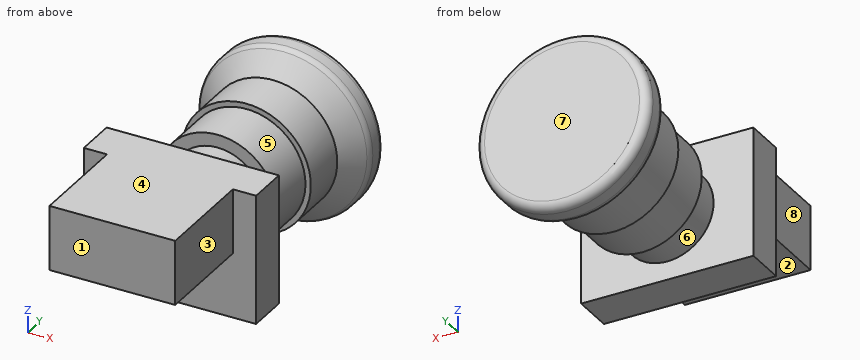
```python
from build123d import *

# Parameters (mm, degrees)
CROQUIS1_W              = 13.75
CROQUIS1_H              = 12
CROQUIS5_R              = 10.75
SALIENTE_EXTRUIR3_DEPTH = 10.3
CROQUIS8_W              = 40
CROQUIS8_H              = 30
SALIENTE_EXTRUIR4_DEPTH = 9.5
CROQUIS9_W              = 29.2
CROQUIS9_H              = 15
SALIENTE_EXTRUIR5_DEPTH = 24


with BuildPart() as part:
    # Croquis1 → Revolución1 (revolve)
    with BuildSketch(Plane.XY, mode=Mode.PRIVATE) as revoluci_n1_sk:
        with Locations((6.875, 6)):
            Rectangle(CROQUIS1_W, CROQUIS1_H)
    revolve(revoluci_n1_sk.sketch.rotate(Axis((0, 0, 0), (0, 1, 0)), 90), axis=Axis((0, 0, 0), (0, 1, 0)))

    # Croquis2 → Revolución2 (revolve)
    with BuildSketch(Plane.XY, mode=Mode.PRIVATE) as revoluci_n2_sk:
        with BuildLine():
            Line((0, 12), (15, 12))
            Line((15, 12), (15, 23))
            Line((15, 23), (19.414213562, 27.414213562))
            ThreePointArc((19.414213562, 27.414213562), (19.847759065, 28.06306026), (20, 28.828427125))
            Line((20, 28.828427125), (20, 31.528143579))
            ThreePointArc((20, 31.528143579), (19.414213562, 32.942357141), (18, 33.528143579))
            Line((18, 33.528143579), (0, 33.528143579))
            Line((0, 33.528143579), (0, 28))
            Line((0, 28), (0, 12))
        make_face()
    revolve(revoluci_n2_sk.sketch.rotate(Axis((0, 28, 0), (0, -1, 0)), 180), axis=Axis((0, 28, 0), (0, -1, 0)))

    # Croquis5 → Saliente-Extruir3 (add)
    with BuildSketch(Plane.XZ):
        with Locations(Location((0, 0, 0), (0, 0, 90))):
            Circle(CROQUIS5_R)
    extrude(amount=SALIENTE_EXTRUIR3_DEPTH)

    # Croquis8 → Saliente-Extruir4 (add)
    with BuildSketch(Plane.XZ.offset(10.3)):
        Rectangle(CROQUIS8_W, CROQUIS8_H)
    extrude(amount=SALIENTE_EXTRUIR4_DEPTH)

    # Croquis9 → Saliente-Extruir5 (add)
    with BuildSketch(Plane.XZ.offset(19.8)):
        with Locations((0, 7.5)):
            Rectangle(CROQUIS9_W, CROQUIS9_H)
    extrude(amount=SALIENTE_EXTRUIR5_DEPTH)


solid = part.part
```
Geometry check sheet. Reference: the model listing, model coordinates, mm. Face numbers are marked on the shaded views. A direction names the side the tool comes from. Give positions to 0.01 mm unless a question says otherwise; leave off trailing zeros. Order: outer loops, then holes, each group sorted by start corner. A loop starts at its lowest first (then second) coordinate and runs counter-clockwise, first axis right, second up.
1. Gauge pin test, flat ends, axial feed: pin 1 Ø3 at (x, z) = (-16, -2.5) entering from -Y; pin 2 Ø8 at (y, z) = (1.5, -9.5) entering from -X; pin 3 Ø3 at (y, z) = (18.5, 0) entering from +X; pin 4 Ø8 at (x, z) = (3, -3) entering from -Y. Record the tip position at first contact, or that the pin passes through.
2. Thickness scan on L1, parallel to Y at x = 4.5, z = 14; L2, parallel to Y at x = -13, z = -6.5; L3, parallel to Z at x = -11, y = -29. Record the ranges inside material, lowest first.
3. Release check for a two-part mould opening along Y. For the marked faces 6, 7 and 8 record: pulls with the +Y half, pulls with the -Y half, needs draft (parallel to the pull), parting line crosses it, or undercut.
4. Section check A-A, the plane x = 0. Enter the section's corners in (y, z).
5. Access from +Z, -Z, +X, -X, +Y, -Y to the whole of each face (thin tool, end or side, straight path). Record for the marked faces 1, 2, 3, 4 and 5.
6. Section check C-C, the plane y = 8.5. Enter the section's corners in (x, z), and give its area (3 significant figures).
7. Section check B-B, the plane y = -26.5. Enter the section's corners in (x, z), and give its area (3 significant figures).
8. Section check D-D, the plane y = 24.5. Enter the section's corners in (x, z), and give its area (3 significant figures).
Values follow:
1. pin 1: stops at y = -19.8
1. pin 2: stops at x = -12.6
1. pin 3: stops at x = 15
1. pin 4: stops at y = -43.8
2. L1: y = -43.8 to -10.3, 12 to 33.53
2. L2: y = -19.8 to -10.3, 12 to 33.53
2. L3: z = 0 to 15
3. face 6: undercut
3. face 7: pulls with the +Y half
3. face 8: needs draft
4. outline: (-43.8, 0) - (-19.8, 0) - (-19.8, -15) - (-10.3, -15) - (-10.3, -10.75) - (0, -10.75) - (0, -13.75) - (12, -13.75) - (12, -15) - (23, -15) - (27.41, -19.41) arc R2 ccw to (28.83, -20) - (31.53, -20) arc R2 ccw to (33.53, -18) - (33.53, 18) arc R2 ccw to (31.53, 20) - (28.83, 20) arc R2 ccw to (27.41, 19.41) - (23, 15) - (12, 15) - (12, 13.75) - (0, 13.75) - (0, 10.75) - (-10.3, 10.75) - (-10.3, 15) - (-43.8, 15) - close
5. face 1: +Z, -Z, +X, -X, -Y
5. face 2: -Z, +X, -X, -Y
5. face 3: +Z, -Z, +X, -Y
5. face 4: +Z, +X, -X, -Y
5. face 5: none
6. outline: circle Ø27.5 at (0, 0)
6. area: 594 mm2
7. outline: (-14.6, 0) - (14.6, 0) - (14.6, 15) - (-14.6, 15) - close
7. area: 438 mm2
8. outline: circle Ø33 at (0, 0)
8. area: 855 mm2
